```python
from build123d import *

# Parameters (mm, degrees)
SKIZZE1_R                        = 31
AUFSATZ_LINEAR_AUSTRAGEN1_DEPTH  = 32
SKIZZE2_W                        = 2.5
SKIZZE2_H                        = 2.15
SCHNITT_LINEAR_AUSTRAGEN1_DEPTH  = 14.5
F_5_5_5_5_DURCHMESSER_BOHRUNG1_D = 5.5
M6_GEWINDEBOHRUNG1_D             = 5
M6_GEWINDEBOHRUNG1_DEPTH         = 17
M6_GEWINDEBOHRUNG1_CSINK_D       = 6.05
M6_GEWINDEBOHRUNG1_CSINK_ANGLE   = 90
M6_GEWINDEBOHRUNG1_TIP           = 1.502151548


with BuildPart() as part:
    # Skizze1 → Aufsatz-Linear austragen1 (new body)
    with BuildSketch(Plane.XY):
        with BuildLine():
            Line((36, 29.103264422), (36, 218))
            ThreePointArc((36, 218), (25.455844123, 243.455844123), (0, 254))
            Line((0, 254), (-43, 254))
            Line((-43, 254), (-43, 0))
            ThreePointArc((-43, 0), (10.055704227, -41.807688438), (38.296875, 19.553755783))
            ThreePointArc((38.296875, 19.553755783), (36.582291693, 24.192339102), (36, 29.103264422))
        make_face()
        Circle(SKIZZE1_R, mode=Mode.SUBTRACT)
        with BuildLine():
            Line((5, 152.5), (-5, 152.5))
            ThreePointArc((-5, 152.5), (-17.5, 165), (-5, 177.5))
            Line((-5, 177.5), (5, 177.5))
            ThreePointArc((5, 177.5), (17.5, 165), (5, 152.5))
        make_face(mode=Mode.SUBTRACT)
    extrude(amount=AUFSATZ_LINEAR_AUSTRAGEN1_DEPTH)

    # Skizze2 → Schnitt-Rotation1 (revolve, cut)
    with BuildSketch(Plane(origin=(0, 0, 0), x_dir=(1, 0, 0), z_dir=(0, 1, 0))):
        with Locations((-31.25, -6.925)):
            Rectangle(SKIZZE2_W, SKIZZE2_H)
        with Locations((-31.25, -25.075)):
            Rectangle(SKIZZE2_W, SKIZZE2_H)
    revolve(axis=Axis((0, 0, 0), (0, 0, 1)), mode=Mode.SUBTRACT)

    # Skizze3 → Schnitt-Linear austragen1 (cut)
    with BuildSketch(Plane.XY.offset(32)):
        with BuildLine():
            Line((-43, 182), (0, 182))
            ThreePointArc((0, 182), (25.455844123, 171.455844123), (36, 146))
            Line((36, 146), (92.796616339, 146))
            Line((92.796616339, 146), (92.796616339, 301.382333193))
            Line((92.796616339, 301.382333193), (-43, 301.382333193))
            Line((-43, 301.382333193), (-43, 182))
        make_face()
    extrude(amount=-SCHNITT_LINEAR_AUSTRAGEN1_DEPTH, mode=Mode.SUBTRACT)

    # Ø5.5 (5.5) Durchmesser Bohrung1 (through all)
    with Locations(Plane.XY.offset(17.5)):
        with Locations((-31.8, 194), (-31.8, 244)):
            Hole(F_5_5_5_5_DURCHMESSER_BOHRUNG1_D / 2)

    # M6 Gewindebohrung1
    with Locations(Plane(origin=(36, 0, -4), x_dir=(0, 0, 1), z_dir=(1, 0, 0))):
        with Locations((26, -134), (26, -119)):
            CounterSinkHole(M6_GEWINDEBOHRUNG1_D / 2, M6_GEWINDEBOHRUNG1_CSINK_D / 2, depth=M6_GEWINDEBOHRUNG1_DEPTH, counter_sink_angle=M6_GEWINDEBOHRUNG1_CSINK_ANGLE)
            with Locations((0, 0, -(M6_GEWINDEBOHRUNG1_DEPTH + M6_GEWINDEBOHRUNG1_TIP / 2))):  # 118° drill point
                Cone(0, M6_GEWINDEBOHRUNG1_D / 2, M6_GEWINDEBOHRUNG1_TIP, mode=Mode.SUBTRACT)


solid = part.part
```
Build history of the part. All positions in model axes, mm. A direction names the side the tool comes from. Coordinates: 2 decimals unless noted, no trailing zeros. Order: outer loops, then holes, each group sorted by start corner. A loop starts at its lowest first (then second) coordinate and runs counter-clockwise, first axis right, second up.
Item 1: Mould opens along Y. For faces 1 (the flat face through (-21, 254, 9)), 2 (the cylindrical face through (-33.07, 241.56, 8.63)), 3 (the flat face through (-10, 141, 0)) say: released by +Y, released by -Y, zero draft, split by the parting line, or undercut.
Filled in:
face 1: released by +Y
face 2: undercut
face 3: zero draft
Item 2: Saw through at C-C on z = 3. List the corners of the cut face in (x, y).
Filled in:
outline: (-43, 0) arc R43 ccw (long way) to (38.3, 19.55) arc R21 cw to (36, 29.1) - (36, 218) arc R36 ccw to (0, 254) - (-43, 254) - close; hole circle Ø5.5 at (-31.8, 194); hole circle Ø5.5 at (-31.8, 244); hole circle Ø62 at (0, 0); hole (-5, 152.5) - (5, 152.5) arc R12.5 ccw to (5, 177.5) - (-5, 177.5) arc R12.5 ccw to start
Item 3: Tool access for faces 4 (the flat face through (-29, 12, 8)), 5 (the flat face through (-22, 182, 25)), 6 (the flat face through (36, 101, 16)), 7 (the cylindrical face through (17.497, 165.275, 15.776)): list every direction of +Z, -Z, +X, -X, +Y, -Y with a clear straight run to the whole face (end or side of a thin tool).
Filled in:
face 4: none
face 5: +Z, +X, -X, +Y
face 6: +Z, -Z, +X, +Y
face 7: +Z, -Z
Item 4: Saw through at B-B on x = -20. List the corners of the cut face in (y, z).
Filled in:
outline: (-38.07, 0) - (-23.69, 0) - (-23.69, 5.85) - (-25.62, 5.85) - (-25.62, 8) - (-23.69, 8) - (-23.69, 24) - (-25.62, 24) - (-25.62, 26.15) - (-23.69, 26.15) - (-23.69, 32) - (-38.07, 32) - close; (23.69, 0) - (254, 0) - (254, 17.5) - (182, 17.5) - (182, 32) - (23.69, 32) - (23.69, 26.15) - (25.62, 26.15) - (25.62, 24) - (23.69, 24) - (23.69, 8) - (25.62, 8) - (25.62, 5.85) - (23.69, 5.85) - close
Item 5: Saw through at A-A on y = 194. List the corners of the cut face in (x, z).
Filled in:
outline: (-43, 0) - (-34.55, 0) - (-34.55, 17.5) - (-43, 17.5) - close; (-29.05, 0) - (36, 0) - (36, 17.5) - (-29.05, 17.5) - close
Item 6: Drop flat-ended pins along their axis: pin 1 Ø1.5 at (y, z) = (8, 8.5) entering from +X; pin 2 Ø6.5 at (x, y) = (-31.8, 194) entering from +Z; pin 3 Ø8 at (x, z) = (-32, 3.5) entering from -Y. Give the stop position or say it passes through.
Filled in:
pin 1: stops at x = 42.38
pin 2: stops at z = 17.5
pin 3: stops at y = -32.63
Item 7: Drill centre lines: L1, parallel to Z at x = -21, y = -24; L2, parallel to Y at x = 0, z = 18.75; L3, parallel to Y at x = 0, z = 16. Where is each one in solid material? Low to high.
Filled in:
L1: z = 0 to 5.85, 8 to 24, 26.15 to 32
L2: y = -43 to -31, 31 to 152.5, 177.5 to 182
L3: y = -43 to -31, 31 to 152.5, 177.5 to 254
Item 8: Saw through at D-D on x = -7.5. State how many separate pieces and enclosed holes the cut face has, then the cut area to 3 significant figures.
Filled in:
separate pieces: 3
enclosed holes: 0
area: 5,720 mm2
